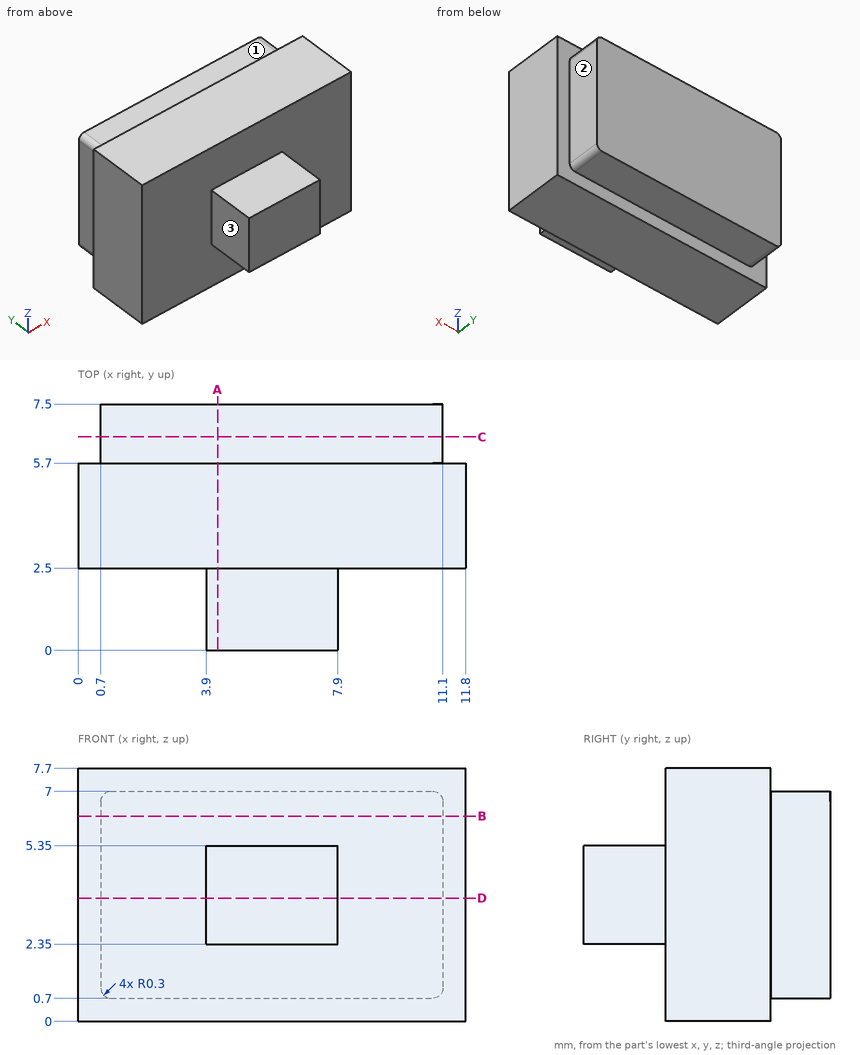
The drawing under review shows one solid part. Ordinate dimensions are in mm from its lowest x, y, z. A direction names the side the tool comes from. Coordinates: 2 decimals unless noted, no trailing zeros. Write each loop counter-clockwise with the first axis right and the second up, starting at its lowest first coordinate (ties: lowest second). Pieces come first, ordered by that corner, then holes.
1) Insertion check: pin 1 (1.4 mm diameter, centred on x = 6.5, y = 6.5, fed in from +Z); pin 2 (0.8 mm diameter, centred on y = 2, z = 4.5, fed in from -X); pin 3 (1.4 mm diameter, centred on y = 7, z = 3.5, fed in from -X). Each pin has a flat end and moves straight along its axis. Give the tip position at first contact, or say it passes through.
2) Add section D-D (z = 3.75). Write out the cut boundary in (x, y).
3) Machinability: for the marked faces 1, 2 and 3, which of the approach directions +Z, -Z, +X, -X, +Y, -Y give a long, thin tool a straight path to every point of the face, cutting with its end or side? Answer none if there is none.
4) Add section A-A (x = 4.25). Write out the cut boundary in (y, z).
5) Add section B-B (z = 6.25). Write out the cut boundary in (x, y).
6) To check wall thickness, follow L1, parallel to X at y = 6.25, z = 6.5; L2, parallel to Y at x = 1, z = 5.25; L3, parallel to Z at x = 3.5, y = 6.5. State the ranges of each line that lie inside material, in increasing order.
7) Add section C-C (y = 6.5). Write out the cut boundary in (x, z), plus the area to 3 significant figures.
Check result:
1. pin 1: stops at z = 7
1. pin 2: stops at x = 3.9
1. pin 3: stops at x = 0.7
2. outline: (0, 2.5) - (3.9, 2.5) - (3.9, 0) - (7.9, 0) - (7.9, 2.5) - (11.8, 2.5) - (11.8, 5.7) - (11.1, 5.7) - (11.1, 7.5) - (0.7, 7.5) - (0.7, 5.7) - (0, 5.7) - close
3. face 1: +Z, +X, -X, +Y
3. face 2: +Z, -Z, +X, +Y
3. face 3: +Z, -Z, -X, -Y
4. outline: (0, 2.35) - (2.5, 2.35) - (2.5, 0) - (5.7, 0) - (5.7, 0.7) - (7.5, 0.7) - (7.5, 7) - (5.7, 7) - (5.7, 7.7) - (2.5, 7.7) - (2.5, 5.35) - (0, 5.35) - close
5. outline: (0, 2.5) - (11.8, 2.5) - (11.8, 5.7) - (11.1, 5.7) - (11.1, 7.5) - (0.7, 7.5) - (0.7, 5.7) - (0, 5.7) - close
6. L1: x = 0.7 to 11.1
6. L2: y = 2.5 to 7.5
6. L3: z = 0.7 to 7
7. outline: (0.7, 1) arc R0.3 ccw to (1, 0.7) - (10.8, 0.7) arc R0.3 ccw to (11.1, 1) - (11.1, 6.7) arc R0.3 ccw to (10.8, 7) - (1, 7) arc R0.3 ccw to (0.7, 6.7) - close
7. area: 65.4 mm2
